from build123d import *

# Parameters (mm, degrees)
BOSS_EXTRUDE2_DEPTH = 21.5
BOSS_EXTRUDE3_DEPTH = 266


with BuildPart() as part:
    # Sketch1 → Boss-Extrude2 (new body)
    with BuildSketch(Plane(origin=(0, 0, 0), x_dir=(1, 0, 0), z_dir=(0, 1, 0))):
        with BuildLine():
            Line((0, 0), (300, 0))
            ThreePointArc((300, 0), (326.870057685, 11.129942315), (338, 38))
            Line((338, 38), (338, 68))
            ThreePointArc((338, 68), (335.071067812, 75.071067812), (328, 78))
            Line((328, 78), (28, 78))
            ThreePointArc((28, 78), (1.129942315, 66.870057685), (-10, 40))
            Line((-10, 40), (-10, 10))
            ThreePointArc((-10, 10), (-7.071067812, 2.928932188), (0, 0))
        make_face()
    extrude(amount=BOSS_EXTRUDE2_DEPTH)

    # Sketch5 → Boss-Extrude3 (add)
    with BuildSketch(Plane(origin=(28, 0, 0), x_dir=(0, 0, -1), z_dir=(1, 0, 0))):
        with BuildLine():
            Line((78, 0), (42, 0))
            Line((42, 0), (42, -8.17))
            Line((42, -8.17), (44.828427125, -10.998427125))
            Line((44.828427125, -10.998427125), (47.658427125, -10.998427125))
            ThreePointArc((47.658427125, -10.998427125), (60, -0.482256494), (72.341572875, -10.998427125))
            Line((72.341572875, -10.998427125), (75.171572875, -10.998427125))
            Line((75.171572875, -10.998427125), (78, -8.17))
            Line((78, -8.17), (78, 0))
        make_face()
    extrude(amount=BOSS_EXTRUDE3_DEPTH)


solid = part.part
Could you check a few things on this model? Use its own coordinates, in mm. A direction names the side the tool comes from. Give positions to 0.01 mm unless a question says otherwise; leave off trailing zeros. Write each loop counter-clockwise with the first axis right and the second up, starting at its lowest first coordinate (ties: lowest second). Pieces come first, ordered by that corner, then holes. Notation, with made-up numbers: (-13.5, 23) - (20.5, 23) arc R15 ccw to (20.5, 38) - close; hole circle Ø8 at (76, 75). An arc over 180 degrees is marked (long way). Use CSV: the item, a comma, the result in double quotes. Start each with the question number.
Item 1: I want a section at C-C, the plane z = -62. Please give me the cut outline in (x, y), then the cut area to 3 significant figures.
Item 2: I want a section at B-B, the plane y = 8. Please give me the cut outline in (x, z), then the cut area to 3 significant figures.
Item 3: I want a section at D-D, the plane z = -17. Please give me the cut outline in (x, y).
Item 4: For faces 1 (the face through (28, -0.5, -55.7)), 2 (the face through (159, -4, -42)), 3 (the face through (294, -0.5, -55.7)), which set-ups out of +Z, -Z, +X, -X, +Y, -Y let a thin tool reach every point of the face, with its end or its side?
Item 5: I'm going to push flat-ended pins straight in: pin 1 (3 mm diameter, centred on y = 6.5, z = -52.5, fed in from -X); pin 2 (9 mm diameter, centred on y = -5, z = -57, fed in from -X); pin 3 (4 mm diameter, centred on x = 194, y = -5, fed in from +Z). Where does each tip first touch, or does it pass through?
Item 6: I want a section at A-A, the plane x = 85. Please give me the cut outline in (y, z), then the cut area to 3 significant figures.
Item 7: If I drill on line 1 along Y through (x, z) = (89, -28); line 2 along Z through (x, y) = (32.5, -8); line 3 along Z through (x, y) = (112.5, -10), over which ranges is the centre line in solid material (lowest first)?
Findings:
1,outline,"(-2.98, 0) - (28, 0) - (28, -0.64) - (294, -0.64) - (294, 0) - (338, 0) - (338, 21.5) - (-2.98, 21.5) - close"
1,area,"7,500 mm2"
2,outline,"(-10, -40) arc R38 ccw to (28, -78) - (328, -78) arc R10 ccw to (338, -68) - (338, -38) arc R38 ccw to (300, 0) - (0, 0) arc R10 ccw to (-10, -10) - close"
2,area,"26,500 mm2"
3,outline,"(-10, 0) - (331.67, 0) - (331.67, 21.5) - (-10, 21.5) - close"
4,face 1,"+Z, -Z, -X, -Y"
4,face 2,"+Z, +X, -X, -Y"
4,face 3,"+Z, -Z, +X, -Y"
5,pin 1,"stops at x = -8.37"
5,pin 2,"stops at x = 28"
5,pin 3,"stops at z = -42"
6,outline,"(-11, -75.17) - (-8.17, -78) - (21.5, -78) - (21.5, 0) - (0, 0) - (0, -42) - (-8.17, -42) - (-11, -44.83) - (-11, -47.66) arc R12.5 cw to (-11, -72.34) - close"
6,area,"1,870 mm2"
7,line 1,"y = 0 to 21.5"
7,line 2,"z = -78 to -71.46, -48.54 to -42"
7,line 3,"z = -76.17 to -72.14, -47.86 to -43.83"
